Autodesk Inventor part; units mm, degrees
ref_plane "Work Plane1" through (0, 0, 25.4) normal (0, 0, -1) x (-1, 0, 0)
ref_plane "Work Plane2" through (0, 0, 31.75) normal (0, 0, -1) x (-1, 0, 0)
ref_plane "Work Plane3" through (0, 0, 44.45) normal (0, 0, -1) x (-1, 0, 0)
sketch "Sketch1" plane through (0, 0, 0) normal (0, 0, 1) x (1, 0, 0)
  circle A0 centre (0, 0) radius 3.937
  dimension "d0" = 7.874
extrude "Extrusion1" add sketch "Sketch1" along normal blind 76.2
sketch "Sketch2" plane through (0, 0, 0) normal (0, 0, -1) x (-1, 0, 0)
  circle A0 centre (0, 0) radius 3.937
  circle A1 centre (0, 0) radius 3.81
  dimension "d3" = 7.62
extrude "Extrusion2" cut sketch "Sketch2" against normal blind 50.8
ref_plane "Work Plane1" through (0, 0, 25.4) normal (0, 0, -1) x (-1, 0, 0)
sketch "Sketch3" plane through (0, 0, 25.4) normal (0, 0, -1) x (-1, 0, 0)
  circle A0 centre (0, 0) radius 3.81
  circle A1 centre (0, 0) radius 1.5875
  dimension "d7" = 3.175
ref_plane "Work Plane2" through (0, 0, 31.75) normal (0, 0, -1) x (-1, 0, 0)
ref_plane "Work Plane3" through (0, 0, 44.45) normal (0, 0, -1) x (-1, 0, 0)
sketch "Sketch4" plane through (0, 0, 31.75) normal (0, 0, -1) x (-1, 0, 0)
  circle A0 centre (0, 0) radius 3.81
  circle A1 centre (0, 0) radius 1.5875
  dimension "d10" = 3.175
sketch "Sketch5" plane through (0, 0, 0) normal (0, 1, 0) x (-1, 0, 0)
  line L0 (3.81, 0) -> (3.81, 50.8)
  line L1 (-3.81, 0) -> (-3.81, 50.8)
  line L2 (5.5118, 31.75) -> (-5.5118, 31.75)
  line L3 (5.5118, 25.4) -> (-5.5118, 25.4)
  line L4 (3.81, 25.4) -> (1.3426, 25.4)
  line L5 (1.3426, 25.4) -> (1.3426, 31.75)
  line L6 (1.3426, 31.75) -> (3.81, 31.75)
  line L7 (3.81, 31.75) -> (3.81, 25.4)
  line L8 (0, 31.75) -> (0, 25.4) construction
revolve "Revolution1" cut sketch "Sketch5" angle 360 about axis through (0, 0, 31.75) along (0, 0, -1) contours L3 L5 L2 L0
sketch "Sketch6" plane through (0, 0, 44.45) normal (0, 0, -1) x (-1, 0, 0)
  circle A0 centre (0, 0) radius 3.81
  circle A1 centre (0, 0) radius 3.937
  line L0 (0, 0) -> (0, 3.81) construction
sketch "Sketch8" plane through (0, 0, 0) normal (1, 0, 0) x (0, 1, 0)
  line L0 (5.5118, 31.75) -> (-5.5118, 31.75)
  line L1 (5.5118, 44.45) -> (-5.5118, 44.45)
  line L2 (1.3249, 31.75) -> (3.8367, 44.45)
  line L3 (0, 31.75) -> (0, 44.45) construction
  line L4 (3.8367, 44.45) -> (3.8367, 31.75)
revolve "Revolution2" cut sketch "Sketch8" angle 360 about axis through (0, 0, 31.75) along (0, 0, 1)
properties part number "transmission plunger"
Geometry check sheet. Reference: the model listing, model coordinates, mm. A direction names the side the tool comes from. Round coordinates to 2 decimals unless told otherwise and drop trailing zeros. Order: outer loops, then holes, each group sorted by start corner. A loop starts at its lowest first (then second) coordinate and runs counter-clockwise, first axis right, second up. Notation, with made-up numbers: (-18, -39.5) - (27, -39.5) arc R12 cw to (27, -30.5) - close; hole circle Ø1 at (24, -31). An arc over 180 degrees is marked (long way). One line per question, with ' | ' between items. Start each with the question number.
(1) Sectioned sample at B-B on z = 54.5. Record the cut outline in (x, y), and give its area (3 significant figures).
(2) Thickness scan on L1, parallel to X at y = -0.25, z = 6; L2, parallel to Y at x = -0.5, z = 16; L3, parallel to X at y = 3.25, z = 69.5. Record the ranges inside material, lowest first. Write a range as [from, to].
(3) Release check for a two-part mould opening along Z. For faces 1 (the cylindrical face through (-0.853, 3.843, 63.322)), 2 (the cylindrical face through (-1.28, -0.4, 28.62)), 3 (the flat face through (0, 0, 76.2)) record: released by +Z, released by -Z, zero draft, split by the parting line, or undercut.
(4) Sectioned sample at D-D on z = 14.5. Record the cut outline in (x, y).
(5) Depth check by flat-ended pin: pin 1 Ø2 at (y, z) = (1.5, 68) entering from -X; pin 2 Ø1 at (x, z) = (-1, 18.5) entering from +Y. Enter the tip coordinate at first touch or a pass-through.
(6) Sectioned sample at A-A on y = 0. Record the cut outline in (x, z) (3 decimals), and give its area (3 significant figures).
(7) Access from +Z, -Z, +X, -X, +Y, -Y to the whole of each face (thin tool, end or side, straight path). Record for faces 4 (the flat face through (0, -2, 25.4)), 5 (the flat face through (0, 0, 0)), 6 (the cylindrical face through (0.83, -3.72, 12.52)).
Conclusion:
1) outline: circle Ø7.87 at (0, 0) | area: 48.7 mm2
2) L1: x = [-3.8, 3.8] | L2: y = [-3.78, 3.78] | L3: x = [-2.22, 2.22]
3) face 1: zero draft | face 2: undercut | face 3: released by +Z
4) outline: circle Ø7.62 at (0, 0)
5) pin 1: stops at x = -3.91 | pin 2: stops at y = 3.78
6) outline: (-3.937, 50.8) - (-3.81, 50.8) - (-3.81, 44.315) - (-1.325, 31.75) - (-1.343, 31.75) - (-1.343, 25.4) - (-3.81, 25.4) - (-3.81, 0) - (3.81, 0) - (3.81, 25.4) - (1.343, 25.4) - (1.343, 31.75) - (1.325, 31.75) - (3.81, 44.315) - (3.81, 50.8) - (3.937, 50.8) - (3.937, 76.2) - (-3.937, 76.2) - close | area: 525 mm2
7) face 4: none | face 5: -Z, +X, -X, +Y, -Y | face 6: -Z
